Source: three-view drawing plus pictorial views. Frame: mm from the lowest corner of the part. Give positions to 0.01 mm unless a question says otherwise; leave off trailing zeros. Loops run counter-clockwise (first coordinate to the right, second up) from the corner with the lowest first, then second, coordinate; pieces in that order, holes last.
1. Section A-A, the plane x = 10. Output: boundary loops of the cut face in (y, z), then the cut area to 3 significant figures.
2. Section B-B, the plane z = 180. Output: boundary loops of the cut face in (x, y).
3. Section C-C, the plane y = 5.75. Output: boundary loops of the cut face in (x, z), then the cut area to 3 significant figures.
4. First-contact query: P1, Ø1, axis at x = 9.5, z = 45.5, coming from the -Y side; P2, Ø3.5, axis at x = 9, z = 95.5, coming from the +Y side; P3, Ø1.5, axis at x = 9, z = 293, coming from the +Y side; P4, Ø6, axis at x = 3.5, z = 216, coming from the -Y side. Flat tips, straight axial feed; report the tip coordinate or a pass-through.
5. Material intervals for line 1 along Y through (x, z) = (10.25, 265); line 2 along X through (y, z) = (17.75, 95) (1 decimal); line 3 along X through (y, z) = (18.5, 35) (1 decimal), sorted ascending.
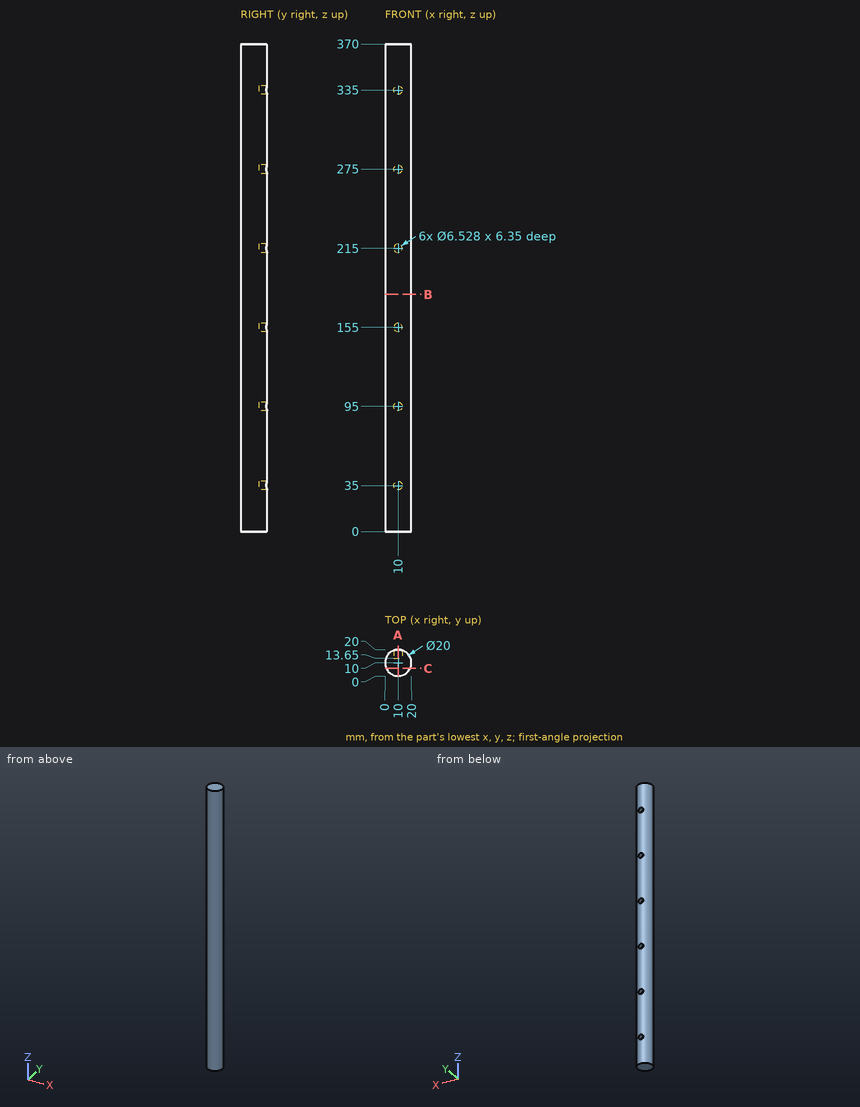
Answers below:
1. outline: (0, 0) - (20, 0) - (20, 31.74) - (13.65, 31.74) - (13.65, 38.26) - (20, 38.26) - (20, 91.74) - (13.65, 91.74) - (13.65, 98.26) - (20, 98.26) - (20, 151.74) - (13.65, 151.74) - (13.65, 158.26) - (20, 158.26) - (20, 211.74) - (13.65, 211.74) - (13.65, 218.26) - (20, 218.26) - (20, 271.74) - (13.65, 271.74) - (13.65, 278.26) - (20, 278.26) - (20, 331.74) - (13.65, 331.74) - (13.65, 338.26) - (20, 338.26) - (20, 370) - (0, 370) - close
1. area: 7,150 mm2
2. outline: circle Ø20 at (10, 10)
3. outline: (0.95, 0) - (19.05, 0) - (19.05, 370) - (0.95, 370) - close
3. area: 6,700 mm2
4. P1: stops at y = 0
4. P2: stops at y = 13.65
4. P3: stops at y = 20
4. P4: stops at y = 0.63
5. line 1: y = 0 to 20
5. line 2: x = 3.7 to 6.7, 13.3 to 16.3
5. line 3: x = 4.7 to 6.7, 13.3 to 15.3
